from build123d import *

# Parameters (mm, degrees)
SKETCH1_R           = 2.25
BOSS_EXTRUDE1_DEPTH = 3
BOSS_EXTRUDE2_DEPTH = 30
BOSS_EXTRUDE3_DEPTH = 30


with BuildPart() as part:
    # Sketch1 → Boss-Extrude1 (new body)
    with BuildSketch(Plane(origin=(0, 0, 0), x_dir=(1, 0, 0), z_dir=(0, 1, 0))):
        Polygon((-7, 23), (-7, -7), (57, -7), (107, -7), (107, 23), (57, 23), align=None)
        with Locations(Location((0, 0, 0), (0, 0, 270))):
            Circle(SKETCH1_R, mode=Mode.SUBTRACT)
        with Locations(Location((0, 16, 0), (0, 0, 270))):
            Circle(SKETCH1_R, mode=Mode.SUBTRACT)
        with Locations(Location((50, 0, 0), (0, 0, 270))):
            Circle(SKETCH1_R, mode=Mode.SUBTRACT)
        with Locations(Location((50, 16, 0), (0, 0, 270))):
            Circle(SKETCH1_R, mode=Mode.SUBTRACT)
    extrude(amount=BOSS_EXTRUDE1_DEPTH)

    # Sketch2 → Boss-Extrude2 (add)
    with BuildSketch(Plane(origin=(0, 0, -23), x_dir=(-1, 0, 0), z_dir=(0, 0, -1))):
        Polygon((7, 3), (7, 20.5), (-7.999999932, 20.5), (-7.999999932, 43.000000035), (-51.999999932, 43.000000035), (-51.999999932, 20.5), (-66.999999864, 20.5), (-66.999999864, 3), (-69.999999864, 3), (-69.999999864, 46.000000035), (-4.999999932, 46.000000035), (-4.999999932, 23.5), (10, 23.5), (10, 0), (7, 0), align=None)
    extrude(amount=-BOSS_EXTRUDE2_DEPTH)

    # Sketch3 → Boss-Extrude3 (add)
    with BuildSketch(Plane(origin=(0, 0, -23), x_dir=(-1, 0, 0), z_dir=(0, 0, -1))):
        Polygon((-4.999999932, 46.000000035), (10, 23.5), (-4.999999932, 23.5), align=None)
    extrude(amount=-BOSS_EXTRUDE3_DEPTH)


solid = part.part
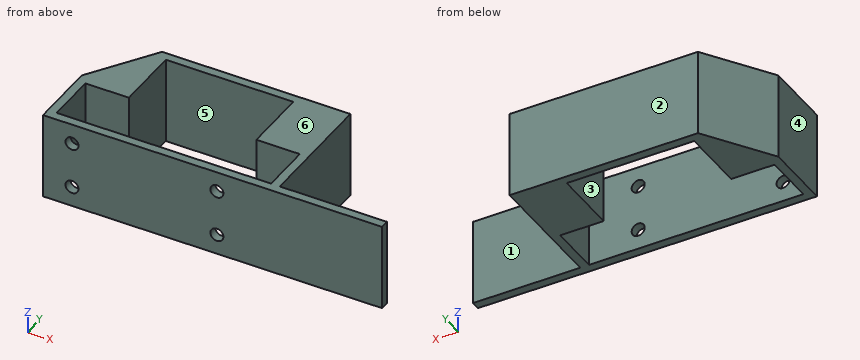
Part model, mm, in its own coordinate system. Face numbers are marked on the shaded views. A direction names the side the tool comes from. Give positions to 0.01 mm unless a question says otherwise; leave off trailing zeros. Write each loop counter-clockwise with the first axis right and the second up, starting at its lowest first coordinate (ties: lowest second). Pieces come first, ordered by that corner, then holes.
1) Two-plate mould, pull along X, no slides. Class the marked faces 4, 5 and 6: released by +X, released by -X, zero draft, split by the parting line, or undercut.
Resolved:
face 4: released by -X
face 5: undercut
face 6: zero draft
2) Probe L1, parallel to X at y = 0.95, z = -16; L2, parallel to X at y = 38.5, z = -10; L3, parallel to X at y = 18, z = 4.5. List the from-to ranges inside material, lowest first.
Resolved:
L1: x = -10 to -2.25, 2.25 to 47.75, 52.25 to 107
L2: x = 0 to 8, 52 to 70
L3: x = -10 to -7, 67 to 70
3) Cut at A-A on z = -16. Write the cut outline in (x, y).
Resolved:
outline: (-10, 0) - (-2.25, 0) - (-2.25, 3) - (-7, 3) - (-7, 20.5) - (8, 20.5) - (8, 43) - (52, 43) - (52, 20.5) - (67, 20.5) - (67, 3) - (52.25, 3) - (52.25, 0) - (107, 0) - (107, 3) - (70, 3) - (70, 46) - (5, 46) - (-10, 23.5) - close; (2.25, 0) - (47.75, 0) - (47.75, 3) - (2.25, 3) - close
4) Pin check, flat tips, straight feed: pin 1 (15 mm diameter, centred on x = 83, z = -10.5, fed in from +Y); pin 2 (5 mm diameter, centred on y = 35, z = -0.5, fed in from +X); pin 3 (2 mm diameter, centred on x = 90, y = 5.5, fed in from -Z); pin 4 (4 mm diameter, centred on x = 0, z = 0, fed in from -Y). Stop position of each tip, or through.
Resolved:
pin 1: stops at y = 3
pin 2: stops at x = 70
pin 3: passes through
pin 4: stops at y = 20.5
5) Cut at C-C on x = 0. Write the cut outline in (y, z).
Resolved:
outline: (0, -23) - (3, -23) - (3, -18.25) - (0, -18.25) - close; (0, -13.75) - (3, -13.75) - (3, -2.25) - (0, -2.25) - close; (0, 2.25) - (3, 2.25) - (3, 7) - (0, 7) - close; (20.5, -23) - (38.5, -23) - (38.5, 7) - (20.5, 7) - close
6) Which spindle directions (+Z, -Z, +X, -X, +Y, -Y) get a long thin tool onto all of the face, cutting with end or side? Do the marked faces 1, 2 and 3. Say none if no direction does.
Resolved:
face 1: +Z, -Z, +X, +Y
face 2: +Z, -Z, +X, -X, +Y
face 3: +Z, -Z
7) Cut at D-D on y = 27. Write the cut outline in (x, z).
Resolved:
outline: (-7.67, -23) - (8, -23) - (8, 7) - (-7.67, 7) - close; (52, -23) - (70, -23) - (70, 7) - (52, 7) - close
8) Cut at B-B on x = 39.5. Write the cut outline in (y, z), then the cut area to 3 significant figures.
Resolved:
outline: (0, -23) - (3, -23) - (3, 7) - (0, 7) - close; (43, -23) - (46, -23) - (46, 7) - (43, 7) - close
area: 180 mm2
